Could you check a few things on this drawing? It's one solid part, dimensions in mm from its lowest x, y, z. A direction names the side the tool comes from. Round coordinates to 2 decimals unless told otherwise and drop trailing zeros. Write each loop counter-clockwise with the first axis right and the second up, starting at its lowest first coordinate (ties: lowest second). Pieces come first, ordered by that corner, then holes. Notation, with made-up numbers: (3.5, -38) - (29.5, -38) arc R28 cw to (29.5, -6) - close; hole circle Ø8 at (52.5, 30.5). An arc over 180 degrees is marked (long way). Use one line per item in the form item = value. Start each with the question number.
1. I want a section at A-A, the plane z = 15. List the corners of the cut face in (x, y) for me, plus the area to 3 significant figures.
2. We'd pull the mould along X, two halves only. Please class the marked faces 3, 4 and 5: +X half, -X half, draft (parallel to the pull), parting line (faces both ways), or undercut.
3. Which directions (+Z, -Z, +X, -X, +Y, -Y) give clear straight access to the entire face, cutting with the end or side of a thin tool? Please do the marked faces 1 and 2.
4. I want a section at C-C, the plane z = 24. List the corners of the cut face in (x, y) for me.
5. Will these pins go through, and if not, where does the flat tip stop? pin 1 (10 mm diameter, centred on x = 15.5, z = 22, fed in from +Y); pin 2 (1.3 mm diameter, centred on y = 7, z = 14, fed in from +X); pin 3 (1 mm diameter, centred on y = 6.5, z = 23, fed in from +X).
6. If I drill on line 1 along Z through (x, y) = (15, 17.25); line 2 along Y through (x, z) = (8, 21.25); line 3 along Z through (x, y) = (26, 15.5), over which ranges is the centre line in solid material (lowest first)?
7. I want a section at B-B, the plane x = 15. List the corners of the cut face in (y, z) for me, plus the area to 3 significant figures.
8. I want a section at D-D, the plane y = 4.25. List the corners of the cut face in (x, z) for me.
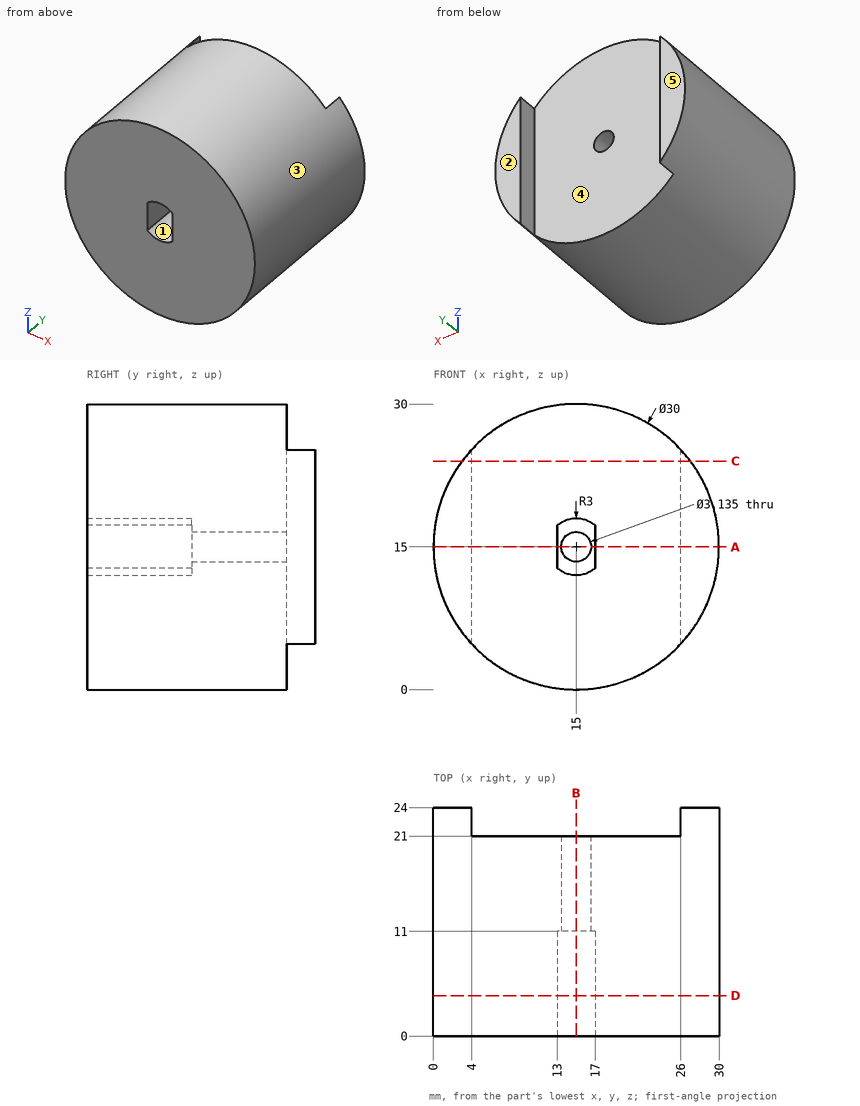
Model answer:
q1.outline = (0, 0) - (13, 0) - (13, 11) - (13.43, 11) - (13.43, 21) - (4, 21) - (4, 24) - (0, 24) - close; (16.57, 11) - (17, 11) - (17, 0) - (30, 0) - (30, 24) - (26, 24) - (26, 21) - (16.57, 21) - close
q1.area = 579 mm2
q2.face_3 = parting line
q2.face_4 = undercut
q2.face_5 = draft
q3.face_1 = -Y
q3.face_2 = +Z, -Z, +X, -X, +Y
q4.outline = (3, 0) - (27, 0) - (27, 24) - (26, 24) - (26, 21) - (4, 21) - (4, 24) - (3, 24) - close
q5.pin_1 = 21
q5.pin_2 = 30
q5.pin_3 = 27.99
q6.line_1 = 0 to 13.43, 16.57 to 30
q6.line_2 = 0 to 21
q6.line_3 = 4.8 to 25.2
q7.outline = (0, 0) - (21, 0) - (21, 13.43) - (11, 13.43) - (11, 12) - (0, 12) - close; (0, 18) - (11, 18) - (11, 16.57) - (21, 16.57) - (21, 30) - (0, 30) - close
q7.area = 533 mm2
q8.outline = circle Ø30 at (15, 15); hole (13, 12.76) arc R3 ccw to (17, 12.76) - (17, 17.24) arc R3 ccw to (13, 17.24) - close
